```python
from build123d import *

# Parameters (mm, degrees)
EXTRUDE_1_DEPTH     = 138.2
EXTRUDE_2_DEPTH     = 52.9
SKETCH_4_R          = 4
CUT_EXTRUDE_1_DEPTH = 12
CHAMFER_1_SIZE      = 1


with BuildPart() as part:
    # 草图1 → 凸台-拉伸1 (new body)
    with BuildSketch(Plane.XY):
        Polygon((-35, 47.5), (35, 47.5), (35, 0), (17, 0), (12, 5), (12, 10.5), (17, 15.5), (17, 21.5), (-17, 21.5), (-17, 15.5), (-12, 10.5), (-12, 5), (-17, 0), (-35, 0), align=None)
    extrude(amount=EXTRUDE_1_DEPTH)

    # 草图2 → 凸台-拉伸2 (add, symmetric)
    with BuildSketch(Plane.XY.offset(69.1)):
        Polygon((-36, 0), (-35, 0), (-35, 47.5), (35, 47.5), (35, 0), (36, 0), (36, 48.5), (15, 48.5), (15, 48), (5, 48), (5, 48.5), (-5, 48.5), (-5, 48), (-15, 48), (-15, 48.5), (-36, 48.5), align=None)
    extrude(amount=EXTRUDE_2_DEPTH, both=True)

    # 草图4 → 切除-拉伸1 (cut)
    with BuildSketch(Plane(origin=(0, 48.5, 0), x_dir=(1, 0, 0), z_dir=(0, 1, 0))):
        with Locations(Location((25, -33.1, 0), (0, 0, 270))):
            Circle(SKETCH_4_R)
        with Locations(Location((25, -105.1, 0), (0, 0, 270))):
            Circle(SKETCH_4_R)
        with Locations(Location((-25, -105.1, 0), (0, 0, 90))):
            Circle(SKETCH_4_R)
        with Locations(Location((-25, -33.1, 0), (0, 0, 90))):
            Circle(SKETCH_4_R)
    extrude(amount=-CUT_EXTRUDE_1_DEPTH, mode=Mode.SUBTRACT)

    # 倒角1
    chamfer_1_edges = [part.edges().sort_by_distance(p)[0] for p in [
        (35, 47.5, 8.1),
        (-35, 47.5, 8.1),
        (35, 0, 8.1),
        (-35, 0, 8.1),
        (36, 0, 69.1),
        (35, 0, 130.1),
        (-35, 0, 130.1),
        (-36, 0, 69.1),
        (36, 48.5, 69.1),
        (-36, 48.5, 69.1),
        (35, 47.5, 130.1),
        (-35, 47.5, 130.1),
    ]]
    chamfer(chamfer_1_edges, length=CHAMFER_1_SIZE - 0.0001)  # a hair under: the kernel refuses the full size


solid = part.part
```
Source: CAD feature listing. Evaluate the final solid. Frame: model axes, mm. A direction names the side the tool comes from. Give positions to 0.01 mm unless a question says otherwise; leave off trailing zeros. Loops run counter-clockwise (first coordinate to the right, second up) from the corner with the lowest first, then second, coordinate; pieces in that order, holes last. Notation, with made-up numbers: (66.5, 0.25) -> (97.5, 0.25) arc R28 ccw to (97.5, 19.25) -> close; hole circle Ø7 at (-21.75, 48). An arc over 180 degrees is marked (long way). Use a Markdown table: item, result. Add a question column.
(1) Access query for faces 4 (the face through (0, 21.5, 68)), 5 (the face through (-25, 36.5, 33)), 6 (the face through (-12, 8, 68)). Directions: +Z, -Z, +X, -X, +Y, -Y. A direction counts if a zero-diameter tool reaches every point of the face in a straight line with its end or side. Return the directions, or none.
(2) Pull-direction query (X, two-part tool) for faces 1 (the face through (10, 48, 70)), 2 (the face through (-35, 23, 8)), 3 (the face through (0, 47.5, 8)); classes: +X half, -X half, draft (parallel to the pull), parting line (faces both ways), or undercut.
(3) Section query B-B (z = 11.5). Output: boundary loops of the cut face in (x, y).
(4) Section query A-A (y = 12). Output: boundary loops of the cut face in (x, z).
(5) Ray query, line 1 (X direction, y = 40, z = 33.1); line 2 (Z direction, x = -25, y = 41.5); line 3 (X direction, y = 19, z = 64.5). Return the intervals inside material, ascending.
(6) Section query C-C (x = -25). Output: boundary loops of the cut face in (y, z).
(7) First-contact query: pin 1 Ø6.5 at (x, z) = (26, 33.5) entering from +Y; pin 2 Ø10 at (x, z) = (5, 63) entering from -Y; pin 3 Ø8 at (x, z) = (8.5, 5.5) entering from +Y; pin 4 Ø3 at (x, z) = (9.5, 84) entering from +Y. Flat tips, straight axial feed; report the tip coordinate or a pass-through.
Checked values:
| question | item | result |
|---|---|---|
| 1 | face 4 | +Z, -Z |
| 1 | face 5 | +Y |
| 1 | face 6 | +Z, -Z, -Y |
| 2 | face 1 | undercut |
| 2 | face 2 | -X half |
| 2 | face 3 | draft |
| 3 | outline | (-35, 1) -> (-34, 0) -> (-17, 0) -> (-12, 5) -> (-12, 10.5) -> (-17, 15.5) -> (-17, 21.5) -> (17, 21.5) -> (17, 15.5) -> (12, 10.5) -> (12, 5) -> (17, 0) -> (34, 0) -> (35, 1) -> (35, 46.5) -> (34, 47.5) -> (-34, 47.5) -> (-35, 46.5) -> close |
| 4 | outline | (-36, 16.2) -> (-35, 16.2) -> (-35, 0) -> (-13.5, 0) -> (-13.5, 138.2) -> (-35, 138.2) -> (-35, 122) -> (-36, 122) -> close; (13.5, 0) -> (35, 0) -> (35, 16.2) -> (36, 16.2) -> (36, 122) -> (35, 122) -> (35, 138.2) -> (13.5, 138.2) -> close |
| 5 | line 1 | -36 to -29, -21 to 21, 29 to 36 |
| 5 | line 2 | 0 to 29.1, 37.1 to 101.1, 109.1 to 138.2 |
| 5 | line 3 | -36 to -17, 17 to 36 |
| 6 | outline | (0, 0) -> (47.5, 0) -> (47.5, 16.2) -> (48.5, 16.2) -> (48.5, 29.1) -> (36.5, 29.1) -> (36.5, 37.1) -> (48.5, 37.1) -> (48.5, 101.1) -> (36.5, 101.1) -> (36.5, 109.1) -> (48.5, 109.1) -> (48.5, 122) -> (47.5, 122) -> (47.5, 138.2) -> (0, 138.2) -> close |
| 7 | pin 1 | y = 48.5 |
| 7 | pin 2 | y = 21.5 |
| 7 | pin 3 | y = 47.5 |
| 7 | pin 4 | y = 48 |
